The drawing under review shows one solid part. Ordinate dimensions are in mm from its lowest x, y, z. A direction names the side the tool comes from. Coordinates: 2 decimals unless noted, no trailing zeros. Order: outer loops, then holes, each group sorted by start corner. A loop starts at its lowest first (then second) coordinate and runs counter-clockwise, first axis right, second up. Notation, with made-up numbers: (41, 30) -> (77, 30) arc R11 ccw to (77, 39) -> close; hole circle Ø2 at (-14.75, -37.75). An arc over 180 degrees is marked (long way). Use one line per item in the form item = value.
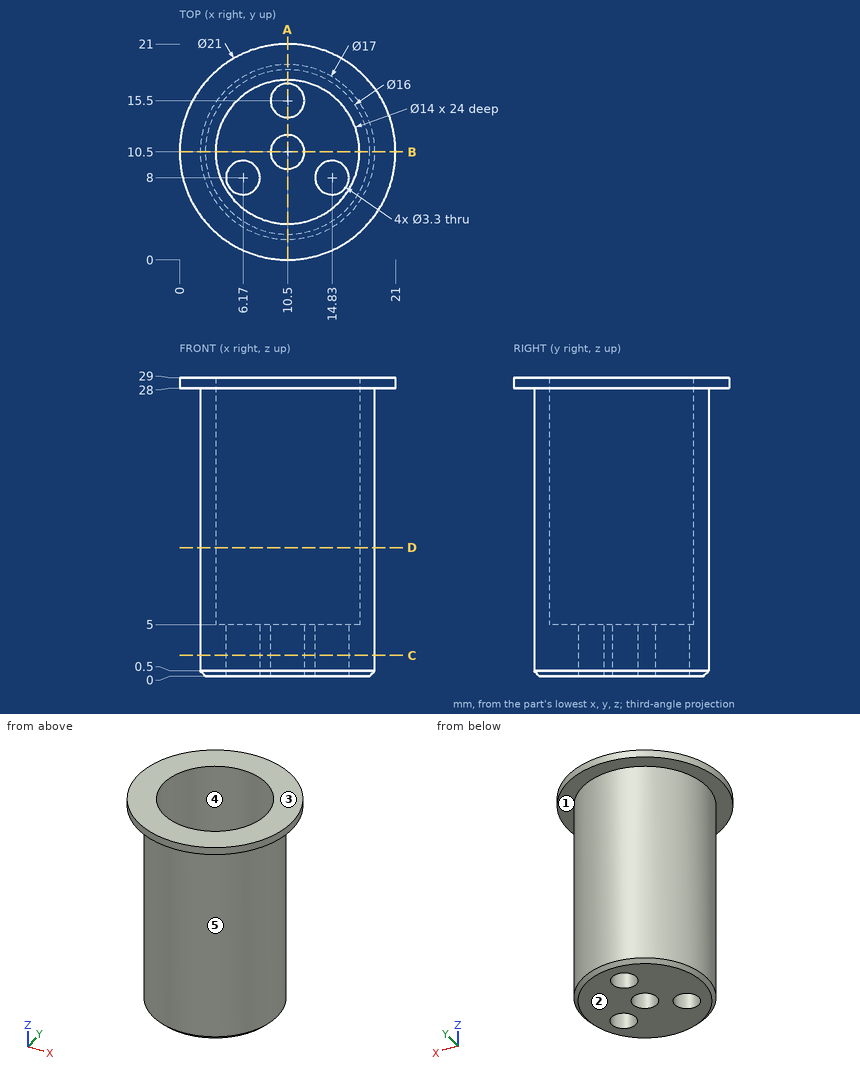
Item 1: To check wall thickness, follow L1, parallel to X at y = 10.25, z = 10.25; L2, parallel to Y at x = 10.5, z = 1.65; L3, parallel to X at y = 8.25, z = 4. State the ranges of each line that lie inside material, in increasing order. Write a range as from..to.
Results found:
L1 = 2..3.5, 17.5..19
L2 = 2..8.85, 12.15..13.85, 17.15..19
L3 = 2.3..4.54, 7.8..13.2, 16.46..18.7
Item 2: We need section B-B (y = 10.5). Write out the cut boundary in (x, z), plus the area to 3 significant figures.
Results found:
outline = (0, 28) -> (2, 28) -> (2, 0.5) -> (2.5, 0) -> (8.85, 0) -> (8.85, 5) -> (3.5, 5) -> (3.5, 29) -> (0, 29) -> close; (12.15, 0) -> (18.5, 0) -> (19, 0.5) -> (19, 28) -> (21, 28) -> (21, 29) -> (17.5, 29) -> (17.5, 5) -> (12.15, 5) -> close
area = 144 mm²
Item 3: We need section D-D (z = 12.5). Write out the cut boundary in (x, y).
Results found:
outline = circle Ø17 at (10.5, 10.5); hole circle Ø14 at (10.5, 10.5)
Item 4: We need section C-C (z = 2). Write out the cut boundary in (x, y).
Results found:
outline = circle Ø17 at (10.5, 10.5); hole circle Ø3.3 at (6.17, 8); hole circle Ø3.3 at (10.5, 10.5); hole circle Ø3.3 at (10.5, 15.5); hole circle Ø3.3 at (14.83, 8)
Item 5: Draft analysis for pull direction Y (two halves, no side actions). For the marked faces 3, 4 and 5, state which applies: released by +Y, released by -Y, zero draft, split by the parting line, or undercut.
Results found:
face_3 = zero draft
face_4 = undercut
face_5 = split by the parting line
Item 6: We need section A-A (x = 10.5). Write out the cut boundary in (y, z), plus the area to 3 significant figures.
Results found:
outline = (0, 28) -> (2, 28) -> (2, 0.5) -> (2.5, 0) -> (8.85, 0) -> (8.85, 5) -> (3.5, 5) -> (3.5, 29) -> (0, 29) -> close; (12.15, 0) -> (13.85, 0) -> (13.85, 5) -> (12.15, 5) -> close; (17.15, 0) -> (18.5, 0) -> (19, 0.5) -> (19, 28) -> (21, 28) -> (21, 29) -> (17.5, 29) -> (17.5, 5) -> (17.15, 5) -> close
area = 128 mm²
Item 7: Clearance check with flat-ended pins moving along their axes: pin 1 (2 mm diameter, centred on y = 3.5, z = 10, fed in from -X); pin 2 (4 mm diameter, centred on y = 6.5, z = 20, fed in from -X); pin 3 (5 mm diameter, centred on y = 17, z = 9.5, fed in from +X). State where each tip first meets the part, or that it passes through.
Results found:
pin_1 = 4.48
pin_2 = 2.24
pin_3 = 18
Item 8: Tool access review of the marked faces 1 and 2: name each direction out of +Z, -Z, +X, -X, +Y, -Y from which nothing blocks a thin tool from reaching the whole face with its end or side.
Results found:
face_1 = -Z
face_2 = -Z, +X, -X, +Y, -Y
